Can you work these out from the model? Positions are in its coordinate system, mm. A direction names the side the tool comes from. Round coordinates to 2 decimals unless told otherwise and drop trailing zeros. Order: outer loops, then holes, each group sorted by start corner. A loop starts at its lowest first (then second) coordinate and runs counter-clockwise, first axis right, second up. Notation, with made-up numbers: (-18.5, 65.25) -> (20.5, 65.25) arc R13 cw to (20.5, 71.25) -> close; hole circle Ø2 at (11, 45.25). An arc over 180 degrees is marked (long way). Use a Markdown table: item, result. Add a question column.
Q1. I'm going to push a flat-ended pin straight in: pin 1 Ø1.5 at (x, y) = (-41, 1.5) entering from -Z. Where does the tip first touch, or does it pass through?
Q2. If we section it at A-A on z = 0: List the corners of the cut face in (x, y) for me, plus the area to 3 significant figures.
Q3. If we section it at B-B on x = 0: List the corners of the cut face in (y, z) for me.
Q4. If we section it at C-C on z = -38: List the corners of the cut face in (x, y) for me.
Q5. We'd pull the mould along Z, two halves only. Please class faces 1 (the face through (-45.728, 1.232, -46.196)), 2 (the face through (-0.459, 1.268, -57.933)), 3 (the face through (-46.196, 1.232, 45.728)): +Z half, -Z half, draft (parallel to the pull), parting line (faces both ways), or undercut.
Q6. If we section it at D-D on x = 60: List the corners of the cut face in (y, z) for me.
Q7. I need wall thicknesses on line 1 along X through (y, z) = (2.35, -14); line 2 along X through (y, z) = (1.2, 54.5). Which ranges of each line are inside material? Lowest first, please. Write a range as [from, to].
Q8. For faces 4 (the face through (-35.18, 1.23, -35.53)), 5 (the face through (45.728, 1.232, 46.196)), which set-ups out of +Z, -Z, +X, -X, +Y, -Y let a thin tool reach every point of the face, with its end or its side?
Autodesk Fusion 360 part; units mm, degrees
sketch "Sketch1" plane through (0, 0, 0) normal (0, 1, 0) x (1, 0, 0)
  circle A0 centre (0, 0) radius 60 construction
  line L0 (-65, -26.9239) -> (-26.9239, -65)
  line L1 (-26.9239, -65) -> (26.9239, -65)
  line L2 (26.9239, -65) -> (65, -26.9239)
  line L3 (65, -26.9239) -> (65, 26.9239)
  line L4 (65, 26.9239) -> (26.9239, 65)
  line L5 (26.9239, 65) -> (-26.9239, 65)
  line L6 (-26.9239, 65) -> (-65, 26.9239)
  line L7 (-65, 26.9239) -> (-65, -26.9239)
  line L8 (-20.7107, -50) -> (20.7107, -50)
  line L9 (20.7107, -50) -> (50, -20.7107)
  line L10 (50, -20.7107) -> (50, 20.7107)
  line L11 (50, 20.7107) -> (20.7107, 50)
  line L12 (20.7107, 50) -> (-20.7107, 50)
  line L13 (-20.7107, 50) -> (-50, 20.7107)
  line L14 (-50, 20.7107) -> (-50, -20.7107)
  line L15 (-50, -20.7107) -> (-20.7107, -50)
  point P0 (-60, 0)
  dimension "d1" = 120
  dimension "d2" = 65
  dimension "d3" = 130
  dimension "d4" = -15
extrude "Extrude1" add sketch "Sketch1" along normal blind 2.5
hole "Hole1" at (-60, 0, 0) direction (0, 1, 0) diameter 4.234 depth 100 tip angle 118
pattern_circular "C-Pattern1" count 16 over 360 about axis through (0, 1.75, 0) along (0, 1, 0) of "Hole1"
fillet "Fillet1" radius 8 16 edges at (-26.9239, 1.25, 65) (26.9239, 1.25, 65) (65, 1.25, 26.9239) (65, 1.25, -26.9239) (26.9239, 1.25, -65) (-26.9239, 1.25, -65) (-65, 1.25, -26.9239) (-65, 1.25, 26.9239) (20.7107, 1.25, -50) (50, 1.25, -20.7107) (50, 1.25, 20.7107) (20.7107, 1.25, 50) (-20.7107, 1.25, 50) (-50, 1.25, 20.7107) (-50, 1.25, -20.7107) (-20.7107, 1.25, -50)
sketch "stage 2 connector clamp cutting pattern" plane through (0, 2.5, 0) normal (0, 1, 0) x (-1, 0, 0)
  arc A0 (65, 23.6102) -> (62.6569, 29.267) centre (57, 23.6102) ccw
  line L0 (62.6569, 29.267) -> (29.267, 62.6569)
  arc A1 (29.267, 62.6569) -> (23.6102, 65) centre (23.6102, 57) ccw
  line L1 (23.6102, 65) -> (-23.6102, 65)
  arc A2 (-23.6102, 65) -> (-29.267, 62.6569) centre (-23.6102, 57) ccw
  line L2 (-29.267, 62.6569) -> (-62.6569, 29.267)
  arc A3 (-62.6569, 29.267) -> (-65, 23.6102) centre (-57, 23.6102) ccw
  line L3 (-65, 23.6102) -> (-65, -23.6102)
  arc A4 (-65, -23.6102) -> (-62.6569, -29.267) centre (-57, -23.6102) ccw
  line L4 (-62.6569, -29.267) -> (-29.267, -62.6569)
  arc A5 (-29.267, -62.6569) -> (-23.6102, -65) centre (-23.6102, -57) ccw
  line L5 (-23.6102, -65) -> (23.6102, -65)
  arc A6 (23.6102, -65) -> (29.267, -62.6569) centre (23.6102, -57) ccw
  line L6 (29.267, -62.6569) -> (62.6569, -29.267)
  arc A7 (62.6569, -29.267) -> (65, -23.6102) centre (57, -23.6102) ccw
  line L7 (65, -23.6102) -> (65, 23.6102)
  circle A8 centre (55.4328, -22.961) radius 2.117
  circle A9 centre (42.4264, -42.4264) radius 2.117
  circle A10 centre (22.961, -55.4328) radius 2.117
  circle A11 centre (0, -60) radius 2.117
  circle A12 centre (-22.961, -55.4328) radius 2.117
  circle A13 centre (-42.4264, -42.4264) radius 2.117
  circle A14 centre (-55.4328, -22.961) radius 2.117
  circle A15 centre (-60, 0) radius 2.117
  circle A16 centre (-55.4328, 22.961) radius 2.117
  circle A17 centre (-42.4264, 42.4264) radius 2.117
  circle A18 centre (-22.961, 55.4328) radius 2.117
  circle A19 centre (0, 60) radius 2.117
  circle A20 centre (22.961, 55.4328) radius 2.117
  circle A21 centre (42.4264, 42.4264) radius 2.117
  circle A22 centre (55.4328, 22.961) radius 2.117
  circle A23 centre (60, 0) radius 2.117
  line L8 (23.0538, 47.6569) -> (47.6569, 23.0538)
  arc A24 (50, 17.397) -> (47.6569, 23.0538) centre (42, 17.397) ccw
  line L9 (50, 17.397) -> (50, -17.397)
  arc A25 (47.6569, -23.0538) -> (50, -17.397) centre (42, -17.397) ccw
  line L10 (47.6569, -23.0538) -> (23.0538, -47.6569)
  arc A26 (17.397, -50) -> (23.0538, -47.6569) centre (17.397, -42) ccw
  line L11 (17.397, -50) -> (-17.397, -50)
  arc A27 (-23.0538, -47.6569) -> (-17.397, -50) centre (-17.397, -42) ccw
  line L12 (-23.0538, -47.6569) -> (-47.6569, -23.0538)
  arc A28 (-50, -17.397) -> (-47.6569, -23.0538) centre (-42, -17.397) ccw
  line L13 (-50, -17.397) -> (-50, 17.397)
  arc A29 (-47.6569, 23.0538) -> (-50, 17.397) centre (-42, 17.397) ccw
  line L14 (-47.6569, 23.0538) -> (-23.0538, 47.6569)
  arc A30 (-17.397, 50) -> (-23.0538, 47.6569) centre (-17.397, 42) ccw
  line L15 (-17.397, 50) -> (17.397, 50)
  arc A31 (23.0538, 47.6569) -> (17.397, 50) centre (17.397, 42) ccw
Answer below:
| question | item | result |
|---|---|---|
| 1 | pin 1 | z = -51.67 |
| 2 | outline | (-65, 0) -> (-62.12, 0) -> (-62.12, 2.5) -> (-65, 2.5) -> close; (-57.88, 0) -> (-50, 0) -> (-50, 2.5) -> (-57.88, 2.5) -> close; (50, 0) -> (57.88, 0) -> (57.88, 2.5) -> (50, 2.5) -> close; (62.12, 0) -> (65, 0) -> (65, 2.5) -> (62.12, 2.5) -> close |
| 2 | area | 53.8 mm² |
| 3 | outline | (0, -65) -> (2.5, -65) -> (2.5, -62.12) -> (0, -62.12) -> close; (0, -57.88) -> (2.5, -57.88) -> (2.5, -50) -> (0, -50) -> close; (0, 50) -> (2.5, 50) -> (2.5, 57.88) -> (0, 57.88) -> close; (0, 62.12) -> (2.5, 62.12) -> (2.5, 65) -> (0, 65) -> close |
| 4 | outline | (-53.92, 0) -> (-32.71, 0) -> (-32.71, 2.5) -> (-53.92, 2.5) -> close; (32.71, 0) -> (53.92, 0) -> (53.92, 2.5) -> (32.71, 2.5) -> close |
| 5 | face 1 | -Z half |
| 5 | face 2 | undercut |
| 5 | face 3 | +Z half |
| 6 | outline | (0, -31.92) -> (2.5, -31.92) -> (2.5, -2.12) -> (0, -2.12) -> close; (0, 2.12) -> (2.5, 2.12) -> (2.5, 31.92) -> (0, 31.92) -> close |
| 7 | line 1 | [-65, -50], [50, 65] |
| 7 | line 2 | [-37.42, -24.86], [-21.06, 21.06], [24.86, 37.42] |
| 8 | face 4 | +Y, -Y |
| 8 | face 5 | +Z, +X, +Y, -Y |
